Input: part model. Units: mm. Frame: model coordinates. A direction names the side the tool comes from. Round coordinates to 2 decimals unless told otherwise and drop trailing zeros. Write each loop counter-clockwise with the first axis right and the second up, starting at its lowest first coordinate (ties: lowest second). Pieces come first, ordered by that corner, then holes. Notation, with made-up numbers: (-9, 8.25) - (46, 8.25) arc R10 cw to (46, 13.25) - close; hole circle Ø6 at (37.25, 29.5). An arc over 180 degrees is marked (long way). Use one line per item in the form item = value.
```python
from build123d import *

# Parameters (mm, degrees)
SKETCH1_R           = 5.588
SKETCH1_R_2         = 2.0828
BOSS_EXTRUDE1_DEPTH = 6.35
BOSS_EXTRUDE2_REACH = 16.016
SKETCH3_R           = 2.0828


with BuildPart() as part:
    # Sketch1 → Boss-Extrude1 (new body)
    with BuildSketch(Plane(origin=(0, 0, 0), x_dir=(1, 0, 0), z_dir=(0, 1, 0))):
        with Locations(Location((0, 0, 0), (0, 0, 270))):
            Circle(SKETCH1_R)
        with Locations(Location((0, 0, 0), (0, 0, 270))):
            Circle(SKETCH1_R_2, mode=Mode.SUBTRACT)
    extrude(amount=BOSS_EXTRUDE1_DEPTH)

    # Sketch3 → Boss-Extrude2 (add, up to next)
    with BuildSketch(Plane(origin=(5.588, 0, 0), x_dir=(0, 0, -1), z_dir=(1, 0, 0)), mode=Mode.PRIVATE) as boss_extrude2_sk1:
        with Locations((0, 3.175)):
            Circle(SKETCH3_R)
    boss_extrude2_tool1 = extrude(boss_extrude2_sk1.sketch, amount=-BOSS_EXTRUDE2_REACH, mode=Mode.PRIVATE) - part.part
    add(boss_extrude2_tool1.solids().sort_by_distance((5.588, 3.175, 0))[0])
    add(boss_extrude2_tool1.solids().sort_by_distance((5.588, 3.175, 0))[1])


solid = part.part
```
(1) Draft query along Z for faces 3 (the face through (5.434, 3.221, 2.082)), 4 (the face through (-5.455, 3.131, -1.211)), 5 (the face through (0.626, 3.131, 1.987)), 6 (the face through (0.1, 0, 2.4)). Return one class per face: released by +Z, released by -Z, zero draft, split by the parting line, or undercut.
Derived:
face_3 = released by +Z
face_4 = split by the parting line
face_5 = undercut
face_6 = zero draft
(2) Cut plane C-C on y = 3. Output: boundary loops of the cut face in (x, z).
Derived:
outline = (5.19, -2.08) - (5.59, -2.08) - (5.59, 2.08) - (5.19, 2.08) arc R5.59 ccw (long way) to start; hole circle Ø4.17 at (0, 0)
(3) Cut plane D-D on x = -1.5. Output: boundary loops of the cut face in (y, z).
Derived:
outline = (0, -5.38) - (6.35, -5.38) - (6.35, -1.45) - (0, -1.45) - close; (0, 1.45) - (6.35, 1.45) - (6.35, 5.38) - (0, 5.38) - close
(4) Cut plane B-B on z = -1.5. Output: boundary loops of the cut face in (x, y).
Derived:
outline = (-5.38, 0) - (-1.45, 0) - (-1.45, 6.35) - (-5.38, 6.35) - close; (1.45, 0) - (5.38, 0) - (5.38, 1.73) - (5.59, 1.73) - (5.59, 4.62) - (5.38, 4.62) - (5.38, 6.35) - (1.45, 6.35) - close
(5) Material intervals for L1, parallel to X at y = 2.5, z = 0; L2, parallel to X at y = 5, z = -1.75; L3, parallel to X at y = 4, z = 3.75, sorted ascending.
Derived:
L1 = -5.59 to -2.08, 2.08 to 5.59
L2 = -5.31 to -1.13, 1.13 to 5.31
L3 = -4.14 to 4.14
(6) Access query for faces 1 (the face through (5.588, 3, 0)), 2 (the face through (5.434, 3.129, -2.082)). Directions: +Z, -Z, +X, -X, +Y, -Y. A direction counts if a zero-diameter tool reaches every point of the face in a straight line with its end or side. Return the directions, or none.
Derived:
face_1 = +Z, -Z, +X, +Y, -Y
face_2 = -Z, +X
(7) Cut plane A-A on x = 0. Output: boundary loops of the cut face in (y, z).
Derived:
outline = (0, -5.59) - (6.35, -5.59) - (6.35, -2.08) - (0, -2.08) - close; (0, 2.08) - (6.35, 2.08) - (6.35, 5.59) - (0, 5.59) - close
(8) First-contact query: pin 1 Ø3 at (y, z) = (4, -2.5) entering from -X. Flat tip, straight axial feed; report the tip coordinate or a pass-through.
Derived:
pin_1 = -5.5
